from build123d import *

# Parameters (mm, degrees)
IZIM2_R                     = 14.63
IZIM2_R_2                   = 1.5
Y_KSEKLIK_EKSTR_ZYON1_DEPTH = 3
KES_EKSTR_ZYON1_START       = -3
KES_EKSTR_ZYON1_DEPTH       = 3
DAIRESEL_KAPLAMA1_COUNT     = 22
IZIM4_R                     = 1.5
Y_KSEKLIK_EKSTR_ZYON2_DEPTH = 3


with BuildPart() as part:
    # Çizim2 → Yükseklik-Ekstrüzyon1 (new body)
    with BuildSketch(Plane(origin=(0, 0, 0), x_dir=(1, 0, 0), z_dir=(0, 1, 0))):
        with Locations(Location((0, 0, 0), (0, 0, 270))):
            Circle(IZIM2_R)
        with Locations(Location((0, 0, 0), (0, 0, 270))):
            Circle(IZIM2_R_2, mode=Mode.SUBTRACT)
    extrude(amount=Y_KSEKLIK_EKSTR_ZYON1_DEPTH)

    # Çizim3 → Kes-Ekstrüzyon1 (cut)
    with BuildSketch(Plane(origin=(0, 3, 0), x_dir=(1, 0, 0), z_dir=(0, 1, 0)).offset(KES_EKSTR_ZYON1_START)):
        with BuildLine():
            ThreePointArc((0.75, 12.066714549), (0, 12.09), (-0.75, 12.066714549))
            ThreePointArc((-0.75, 12.066714549), (-0.963393925, 13.412425983), (-1.75, 14.524957831))
            ThreePointArc((-1.75, 14.524957831), (0, 14.63), (1.75, 14.524957831))
            ThreePointArc((1.75, 14.524957831), (0.963393925, 13.412425983), (0.75, 12.066714549))
        make_face()
    kes_ekstr_zyon1 = extrude(amount=KES_EKSTR_ZYON1_DEPTH, mode=Mode.SUBTRACT)

    # Dairesel Kaplama1: Kes-Ekstrüzyon1 ×22 about axis
    dairesel_kaplama1_axis = Axis((0, 0, 0), (0, 1, 0))
    for i in range(1, DAIRESEL_KAPLAMA1_COUNT):
        add(kes_ekstr_zyon1.rotate(dairesel_kaplama1_axis, i * 360 / DAIRESEL_KAPLAMA1_COUNT), mode=Mode.SUBTRACT)

    # Çizim4 → Yükseklik-Ekstrüzyon2 (add)
    with BuildSketch(Plane(origin=(0, 3, 0), x_dir=(1, 0, 0), z_dir=(0, 1, 0))):
        with BuildLine():
            Line((31, 4), (4.554699728, 4))
            Line((4.554699728, 4), (4.554699728, -4))
            Line((4.554699728, -4), (31, -4))
            ThreePointArc((31, -4), (35, 0), (31, 4))
        make_face()
        with Locations(Location((31, 0, 0), (0, 0, 270))):
            Circle(IZIM4_R, mode=Mode.SUBTRACT)
    extrude(amount=-Y_KSEKLIK_EKSTR_ZYON2_DEPTH)


solid = part.part
For this review, take the finished solid that the model builds, in its own axes (mm). Round coordinates to 2 decimals unless told otherwise and drop trailing zeros. Loops run counter-clockwise (first coordinate to the right, second up) from the corner with the lowest first, then second, coordinate; pieces in that order, holes last. Notation, with made-up numbers: (76.5, 88) - (94.5, 88) arc R5 ccw to (94.5, 92) - close; hole circle Ø5 at (30, -2.5). An arc over 180 degrees is marked (long way). Use one line per item in the form item = value.
1) Wall thickness on probe 1 along X at (y, z) = (0.65, 0); probe 2 along X at (y, z) = (1.65, -12.5); probe 3 along Z at (x, y) = (-6, 2.85): over which ranges is each line inside the solid? List them lowest first.
Solutions:
probe_1 = -14.63 to -1.5, 1.5 to 29.5, 32.5 to 35
probe_2 = -6.49 to -4.63, -2.85 to -0.75, 0.75 to 2.85, 4.63 to 6.49
probe_3 = -13.34 to -10.71, -10.5 to 10.5, 10.71 to 13.34
2) We need section B-B on y = 1.25. State how many separate pieces and enclosed holes the cut face has, then the cut area to 3 significant figures.
Solutions:
separate_pieces = 1
enclosed_holes = 2
area = 711 mm2
3) Clearance check with flat-ended pins moving along their axes: P1, Ø1.5, axis at x = 19.5, y = 1.5, coming from the +Z side; P2, Ø1, axis at x = 29, y = 0.5, coming from the -Z side. State where each tip first meets the part, or that it passes through.
Solutions:
P1 = 4
P2 = -4
4) We need section A-A on x = 0. Write out the cut boundary in (y, z).
Solutions:
outline = (0, -12.09) - (3, -12.09) - (3, -1.5) - (0, -1.5) - close; (0, 1.5) - (3, 1.5) - (3, 12.09) - (0, 12.09) - close
5) We need section C-C on x = 8. Write out the cut boundary in (y, z), then the cut area to 3 significant figures.
Solutions:
outline = (0, -10.72) - (3, -10.72) - (3, 10.72) - (0, 10.72) - close
area = 64.3 mm2
6) Mouldability with a two-part tool opening along Z and no side actions: class faces 1 (the face through (23, 2, -4)), 2 (the face through (-12.581, 1.479, -4.695)), 3 (the face through (-12.62, 1.479, 4.696)) as pulls with the +Z half, pulls with the -Z half, needs draft (parallel to the pull), parting line crosses it, or undercut.
Solutions:
face_1 = pulls with the -Z half
face_2 = undercut
face_3 = undercut
